from build123d import *

# Parameters (mm, degrees)
SKETCH1_W               = 101.6
SKETCH1_H               = 101.6
BOSS_EXTRUDE1_DEPTH     = 19.05
SKETCH2_R               = 3.4925
CUT_EXTRUDE1_DEPTH      = 1
CUT_EXTRUDE1_DEPTH_BACK = 20.05


with BuildPart() as part:
    # Sketch1 → Boss-Extrude1 (new body)
    with BuildSketch(Plane(origin=(0, 0, 0), x_dir=(1, 0, 0), z_dir=(0, 1, 0))):
        Rectangle(SKETCH1_W, SKETCH1_H)
    extrude(amount=BOSS_EXTRUDE1_DEPTH)

    # Sketch2 → Cut-Extrude1 (cut, two sides)
    with BuildSketch(Plane(origin=(0, 19.05, 0), x_dir=(1, 0, 0), z_dir=(0, 1, 0))) as cut_extrude1_sk:
        Circle(SKETCH2_R)
    extrude(amount=CUT_EXTRUDE1_DEPTH, mode=Mode.SUBTRACT)
    extrude(cut_extrude1_sk.sketch, amount=-CUT_EXTRUDE1_DEPTH_BACK, mode=Mode.SUBTRACT)


solid = part.part
Verification items for the finished model (mm, model axes). Coordinates: 2 decimals unless noted, no trailing zeros. Order: outer loops, then holes, each group sorted by start corner. A loop starts at its lowest first (then second) coordinate and runs counter-clockwise, first axis right, second up. Notation, with made-up numbers: (-0.75, -19.75) -> (31.25, -19.75) arc R18 cw to (31.25, 15.25) -> close; hole circle Ø7 at (-28, 42). An arc over 180 degrees is marked (long way). Put each result on its own line as item: value. Start each with the question number.
1. Material ranges on L1, parallel to Z at x = 0, y = 5, recorded low to high. Write a range as [from, to].
2. Cross-section at A-A, the plane x = 0. Record the boundary of the cut face in (y, z), then the cut area to 3 significant figures.
3. Mould release check, pull along Z, two halves, no side actions. Record for faces 1 (the flat face through (-1, 9, -50.8)), 2 (the flat face through (11, 0, -1)), 3 (the cylindrical face through (-0.455, 9.658, -3.463)), 4 (the flat face through (-1, 9, 50.8)): released by +Z, released by -Z, zero draft, split by the parting line, or undercut.
4. Cross-section at B-B, the plane z = 0. Record the boundary of the cut face in (x, y), then the cut area to 3 significant figures.
Computed:
1. L1: [-50.8, -3.49], [3.49, 50.8]
2. outline: (0, -50.8) -> (19.05, -50.8) -> (19.05, -3.49) -> (0, -3.49) -> close; (0, 3.49) -> (19.05, 3.49) -> (19.05, 50.8) -> (0, 50.8) -> close
2. area: 1,800 mm2
3. face 1: released by -Z
3. face 2: zero draft
3. face 3: undercut
3. face 4: released by +Z
4. outline: (-50.8, 0) -> (-3.49, 0) -> (-3.49, 19.05) -> (-50.8, 19.05) -> close; (3.49, 0) -> (50.8, 0) -> (50.8, 19.05) -> (3.49, 19.05) -> close
4. area: 1,800 mm2
